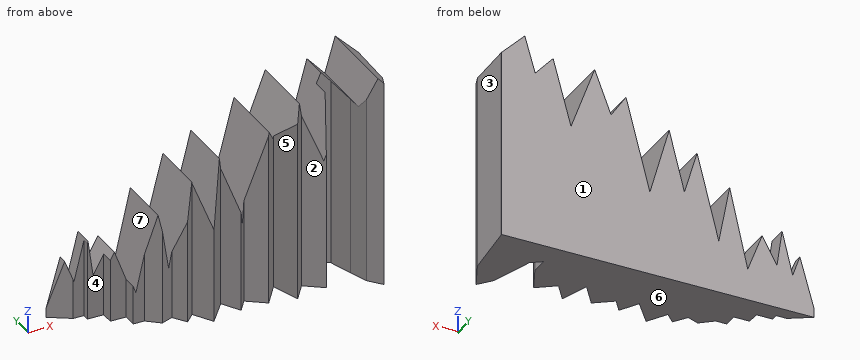
```python
from build123d import *

# Parameters (mm, degrees)
F2_DEPTH = 188.468
F3_DEPTH = 66.595839


with BuildPart() as f2:
    # F1 (on Top) → F2 (new body)
    with BuildSketch(Plane.XY):
        Polygon((238.254488, 0), (0, 0), (15.567613, -9.763042), (23.834057, -9.763042), (23.834057, -14.92957), (36.233719, -14.92957), (36.233719, -24.573755), (48.288953, -24.573755), (48.288953, -34.906808), (56.899831, -34.906808), (66.544011, -42.828817), (75.499326, -39.384466), (82.388029, -49.373083), (89.621171, -42.139944), (98.576479, -56.950655), (113.38719, -38.35116), (121.653639, -52.473001), (128.886774, -42.48438), (142.680591, -52.473001), (155.400931, -34.906808), (162.641421, -56.606222), (172.867577, -42.48438), (186.661394, -52.473001), (196.396053, -31.806894), (196.396053, -18.718356), (204.482083, -24.573755), (210.173458, -42.48438), (214.995548, -56.606222), (223.261997, -66.594839), (233.683616, -44.470357), align=None)
    extrude(amount=F2_DEPTH)

    # F0 (on Front) → F3 (intersect, through all)
    with BuildSketch(Plane.XZ):
        Polygon((10.664172, 44.642482), (0, 7.384356), (0, 0), (238.133401, 0), (238.133401, 143.988803), (220.514372, 161.607817), (212.585822, 134.434521), (198.931083, 149.714991), (185.276344, 99.941269), (167.216852, 149.714991), (154.719889, 117.364436), (143.336907, 134.434521), (125.075892, 64.566277), (110.387675, 117.364436), (98.749742, 71.781114), (89.090228, 105.129436), (72.531059, 40.272702), (64.251475, 84.66047), (50.452169, 24.173511), (39.412726, 53.612031), (28.14329, 33.37305), (24.23349, 61.201647), (16.183894, 28.77328), align=None)
    extrude(amount=F3_DEPTH, mode=Mode.INTERSECT)


solid = f2.part
```
Input: part model. Units: mm. Frame: model coordinates. Face numbers are marked on the shaded views. A direction names the side the tool comes from. Give positions to 0.01 mm unless a question says otherwise; leave off trailing zeros. Order: outer loops, then holes, each group sorted by start corner. A loop starts at its lowest first (then second) coordinate and runs counter-clockwise, first axis right, second up. Notation, with made-up numbers: M -31.75,65 L 3.25,65 A5 ccw 3.25,72 Z; hole C 67.5,81 d8. An arc over 180 degrees is marked long. One line per question, with ' | ' between items.
1) Section B-B on x = 42. Output: boundary loops of the cut face in (y, z).
Filled in:
outline: M -24.57,0 L 0,0 L 0,46.71 L -24.57,46.71 Z
2) Contact query for flat-ended pins moving along their axis: P1, Ø3, axis at y = -28, z = 16.5, coming from the -X side; P2, Ø3.5, axis at x = 29.5, z = 26, coming from the -Y side; P3, Ø6, axis at y = -25, z = 24.5, coming from the +X side; P4, Ø3, axis at x = 177, z = 128.5, coming from the +Y side. Output: stop coordinate, or through.
Filled in:
P1: stops at x = 48.29 | P2: stops at y = -14.93 | P3: stops at x = 235.99 | P4: passes through
3) Ray query, L1, parallel to X at y = -32, z = 86.5; L2, parallel to X at y = -13, z = 144.5; L3, parallel to X at y = -17, z = 109. Return the intervals inside material, ascending.
Filled in:
L1: x = 84.33 to 94.49, 102.51 to 118.97, 130.81 to 196.31, 206.84 to 234.97 | L2: x = 165.2 to 169.11, 197.5 to 203.59, 215.52 to 236.92 | L3: x = 108.25 to 112.71, 136.69 to 181.99, 187.76 to 236.51
4) Section A-A on x = 92. Output: boundary loops of the cut face in (y, z).
Filled in:
outline: M -46.07,0 L 0,0 L 0,95.08 L -46.07,95.08 Z
5) Access query for the marked faces 4, 5, 6 and 7. Directions: +Z, -Z, +X, -X, +Y, -Y. A direction counts if a zero-diameter tool reaches every point of the face in a straight line with its end or side. Return the directions, or none.
Filled in:
face 4: +Z, -Z, -X, -Y | face 5: +Z, -Z, -Y | face 6: -Z, +X, -X, +Y, -Y | face 7: +Z, +Y, -Y
6) Draft query along X for the marked faces 1, 2 and 3. Return one class per face: pulls with the +X half, pulls with the -X half, needs draft (parallel to the pull), parting line crosses it, or undercut.
Filled in:
face 1: needs draft | face 2: undercut | face 3: pulls with the +X half
